from build123d import *

# Parameters (mm, degrees)
SKETCH1_W           = 1208
SKETCH1_H           = 387
BOSS_EXTRUDE1_DEPTH = 4
SKETCH2_W           = 1200
SKETCH2_H           = 604
BOSS_EXTRUDE2_DEPTH = 375
SKETCH3_W           = 158
SKETCH3_H           = 596
SKETCH3_W_2         = 910
SKETCH3_W_3         = 116
CUT_EXTRUDE1_DEPTH  = 371


with BuildPart() as part:
    # Sketch1 → Boss-Extrude1 (new body)
    with BuildSketch(Plane.XY):
        Rectangle(SKETCH1_W, SKETCH1_H)
    extrude(amount=BOSS_EXTRUDE1_DEPTH)

    # Sketch2 → Boss-Extrude2 (add)
    with BuildSketch(Plane(origin=(0, -187.5, 0), x_dir=(1, 0, 0), z_dir=(0, 1, 0))):
        with Locations((0, 302)):
            Rectangle(SKETCH2_W, SKETCH2_H)
    extrude(amount=BOSS_EXTRUDE2_DEPTH)

    # Sketch3 → Cut-Extrude1 (cut)
    with BuildSketch(Plane(origin=(0, 187.5, 0), x_dir=(1, 0, 0), z_dir=(0, 1, 0))):
        with Locations((-517, 302)):
            Rectangle(SKETCH3_W, SKETCH3_H)
        with Locations((21, 302)):
            Rectangle(SKETCH3_W_2, SKETCH3_H)
        with Locations((538, 302)):
            Rectangle(SKETCH3_W_3, SKETCH3_H)
    extrude(amount=-CUT_EXTRUDE1_DEPTH, mode=Mode.SUBTRACT)


solid = part.part
Build history of the part. All positions in model axes, mm. A direction names the side the tool comes from. Round coordinates to 2 decimals unless told otherwise and drop trailing zeros. Loops run counter-clockwise (first coordinate to the right, second up) from the corner with the lowest first, then second, coordinate; pieces in that order, holes last. Notation, with made-up numbers: (3, 29.5) -> (57, 29.5) arc R25 ccw to (57, 58.5) -> close; hole circle Ø4 at (33.25, 3). An arc over 180 degrees is marked (long way). Use CSV: the item, a comma, the result in double quotes. Start each with the question number.
Q1. Saw through at A-A on y = 77.5. Give the cut face in (x, z).
Q2. Saw through at C-C on x = 459. Give the cut face in (y, z).
Q3. Mould opens along Z. For faces 4 (the face through (-518, -183.5, -306)), 5 (the face through (-600, -3, -298)), 6 (the face through (-8, -3, -604)) say: +Z half, -Z half, draft (parallel to the pull), parting line (faces both ways), or undercut.
Q4. Saw through at B-B on z = -493. Give the cut face in (x, y), and give its area (3 significant figures).
Q5. Which spindle directions (+Z, -Z, +X, -X, +Y, -Y) get a long thin tool onto all of the face, cutting with end or side? Do faces 1 (the face through (-8, -187.5, -306)), 2 (the face through (600, -3, -298)), 3 (the face through (596, 5, -298)). Say none if no direction does.
Q6. Drill centre lines: L1, parallel to X at y = 91, z = -415; L2, parallel to Z at x = 516, y = 8; L3, parallel to Y at x = -492.5, z = -149. Where is each one in solid material? Low to high.
Q7. Flat gauge pins, fed straight in: pin 1 Ø6 at (y, z) = (-19, -472) entering from +X; pin 2 Ø4 at (x, z) = (-277.5, -347) entering from -Y; pin 3 Ø5 at (y, z) = (-134, -189.5) entering from -X. Where does each tip first touch, or does it go through?
Solutions:
1,outline,"(-604, 0) -> (-600, 0) -> (-600, -604) -> (600, -604) -> (600, 0) -> (604, 0) -> (604, 4) -> (-604, 4) -> close; hole (-596, -600) -> (-438, -600) -> (-438, -4) -> (-596, -4) -> close; hole (-434, -600) -> (476, -600) -> (476, -4) -> (-434, -4) -> close; hole (480, -600) -> (596, -600) -> (596, -4) -> (480, -4) -> close"
2,outline,"(-193.5, 0) -> (-187.5, 0) -> (-187.5, -604) -> (187.5, -604) -> (187.5, -600) -> (-183.5, -600) -> (-183.5, -4) -> (187.5, -4) -> (187.5, 0) -> (193.5, 0) -> (193.5, 4) -> (-193.5, 4) -> close"
3,face 4,"undercut"
3,face 5,"draft"
3,face 6,"-Z half"
4,outline,"(-600, -187.5) -> (600, -187.5) -> (600, 187.5) -> (596, 187.5) -> (596, -183.5) -> (480, -183.5) -> (480, 187.5) -> (476, 187.5) -> (476, -183.5) -> (-434, -183.5) -> (-434, 187.5) -> (-438, 187.5) -> (-438, -183.5) -> (-596, -183.5) -> (-596, 187.5) -> (-600, 187.5) -> close"
4,area,"10,700 mm^2"
5,face 1,"-Z, +X, -X, -Y"
5,face 2,"-Z, +X, +Y, -Y"
5,face 3,"+Y"
6,L1,"x = -600 to -596, -438 to -434, 476 to 480, 596 to 600"
6,L2,"z = -604 to -600, -4 to 4"
6,L3,"y = -187.5 to -183.5"
7,pin 1,"stops at x = 600"
7,pin 2,"stops at y = -187.5"
7,pin 3,"stops at x = -600"
